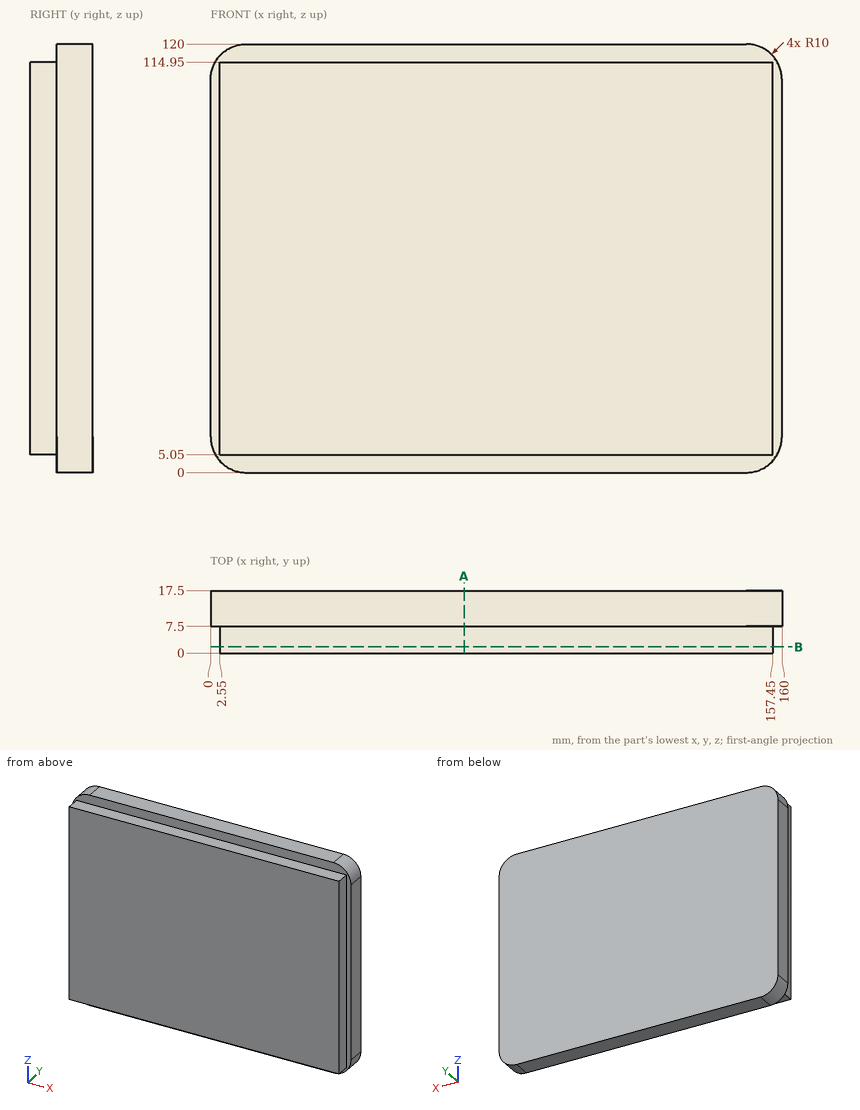
Study the drawing (mm; zero at the part's minimum x, y, z) and answer. Round coordinates to 2 decimals unless told otherwise and drop trailing zeros. Loops run counter-clockwise (first coordinate to the right, second up) from the corner with the lowest first, then second, coordinate; pieces in that order, holes last. Notation, with made-up numbers: M 9.25,22.5 L 21.25,22.5 A20 cw 21.25,34.5 Z; hole C 64,-3 d2. An arc over 180 degrees is marked long. One line per question, with ' | ' between items.
Q1. Consider line 1 along Z through (x, y) = (12, 3.5); line 2 along X through (y, z) = (6.25, 110). Determine where each line is inside the solid, lowest interval first. Write a range as from..to.
Conclusion:
line 1: z = 5.05..114.95 | line 2: x = 2.55..157.45
Q2. Each of these flat-tipped pins is pushed along its axis until it touches: pin 1 Ø1 at (y, z) = (2.5, 98) entering from -X; pin 2 Ø1 at (x, y) = (92, 5.5) entering from +Z; pin 3 Ø8 at (x, y) = (108.5, 2.5) entering from -Z. Where does it stop, or does it pass through?
Conclusion:
pin 1: stops at x = 2.55 | pin 2: stops at z = 114.95 | pin 3: stops at z = 5.05
Q3. Find section B-B, the plane y = 1.75. Give the vertices of the cut face in (x, z), then the cut area to 3 significant figures.
Conclusion:
outline: M 2.55,5.05 L 157.45,5.05 L 157.45,114.95 L 2.55,114.95 Z | area: 17,000 mm2
Q4. Find section A-A, the plane x = 71. Give the vertices of the cut face in (y, z), then the cut area to 3 significant figures.
Conclusion:
outline: M 0,5.05 L 7.5,5.05 L 7.5,0 L 17.5,0 L 17.5,120 L 7.5,120 L 7.5,114.95 L 0,114.95 Z | area: 2,020 mm2
